from build123d import *

# Parameters (mm, degrees)
F1_DEPTH = 3


with BuildPart() as f1:
    # F0 (on Top) → F1 (new body)
    with BuildSketch(Plane.XY):
        Polygon((-34.93066, -38.541029), (-34.93066, 10.958971), (-52.43066, 10.958971), (-52.43066, 13.958971), (-67.43066, 13.958971), (-67.43066, 10.958971), (-84.93066, 10.958971), (-84.93066, -38.541029), (-87.93066, -38.541029), (-87.93066, -48.541029), (-84.93066, -48.541029), (-84.93066, -53.541029), (-82.93066, -53.541029), (-82.93066, -52.041029), (-80.43066, -52.041029), (-80.43066, -53.541029), (-77.43066, -53.541029), (-77.43066, -56.541029), (-80.43066, -56.541029), (-80.43066, -58.041029), (-82.93066, -58.041029), (-82.93066, -56.541029), (-84.93066, -56.541029), (-84.93066, -61.541029), (-87.93066, -61.541029), (-87.93066, -71.541029), (-84.93066, -71.541029), (-84.93066, -121.041029), (-67.43066, -121.041029), (-67.43066, -124.041029), (-52.43066, -124.041029), (-52.43066, -121.041029), (-34.93066, -121.041029), (-34.93066, -71.541029), (-31.93066, -71.541029), (-31.93066, -61.541029), (-34.93066, -61.541029), (-34.93066, -56.541029), (-36.93066, -56.541029), (-36.93066, -58.041029), (-39.43066, -58.041029), (-39.43066, -56.541029), (-42.43066, -56.541029), (-42.43066, -53.541029), (-39.43066, -53.541029), (-39.43066, -52.041029), (-36.93066, -52.041029), (-36.93066, -53.541029), (-34.93066, -53.541029), (-34.93066, -48.541029), (-31.93066, -48.541029), (-31.93066, -38.541029), align=None)
        with BuildLine():
            Line((-75.93066, -81.041029), (-43.93066, -81.041029))
            ThreePointArc((-43.93066, -81.041029), (-42.869999, -81.480369), (-42.43066, -82.541029))
            Line((-42.43066, -82.541029), (-42.43066, -109.541029))
            ThreePointArc((-42.43066, -109.541029), (-42.869999, -110.601689), (-43.93066, -111.041029))
            Line((-43.93066, -111.041029), (-75.93066, -111.041029))
            ThreePointArc((-75.93066, -111.041029), (-76.99132, -110.601689), (-77.43066, -109.541029))
            Line((-77.43066, -109.541029), (-77.43066, -82.541029))
            ThreePointArc((-77.43066, -82.541029), (-76.99132, -81.480369), (-75.93066, -81.041029))
        make_face(mode=Mode.SUBTRACT)
        with BuildLine():
            ThreePointArc((-77.43066, -0.541029), (-76.99132, 0.519631), (-75.93066, 0.958971))
            Line((-75.93066, 0.958971), (-43.93066, 0.958971))
            ThreePointArc((-43.93066, 0.958971), (-42.869999, 0.519631), (-42.43066, -0.541029))
            Line((-42.43066, -0.541029), (-42.43066, -27.541029))
            ThreePointArc((-42.43066, -27.541029), (-42.869999, -28.601689), (-43.93066, -29.041029))
            Line((-43.93066, -29.041029), (-75.93066, -29.041029))
            ThreePointArc((-75.93066, -29.041029), (-76.99132, -28.601689), (-77.43066, -27.541029))
            Line((-77.43066, -27.541029), (-77.43066, -0.541029))
        make_face(mode=Mode.SUBTRACT)
    extrude(amount=F1_DEPTH)


solid = f1.part
The model under review builds one solid part; all positions refer to its coordinate system, in mm. A direction names the side the tool comes from. Give positions to 0.01 mm unless a question says otherwise; leave off trailing zeros. Order: outer loops, then holes, each group sorted by start corner. A loop starts at its lowest first (then second) coordinate and runs counter-clockwise, first axis right, second up. Notation, with made-up numbers: M -29,18.5 L 1,18.5 A26 ccw 1,50.5 Z; hole C 34.25,45.25 d1. An arc over 180 degrees is marked long. Use one line per item in the form item = value. Start each with the question number.
Item 1: We need section D-D on z = 1.4. Give the number of separate pieces and of enclosed holes in the cut face, plus the area to 3 significant figures.
Item 2: To check wall thickness, follow line 1 along Y through (x, z) = (-51.5, 0.8); line 2 along Y through (x, z) = (-58.5, 1.8); line 3 along X through (y, z) = (-100.5, 2.4). State the ranges of each line that lie inside material, in increasing order. Write a range as from..to.
Item 3: We need section B-B on x = -74. Give the boundary of the cut face in (y, z), plus the area to 3 significant figures.
Item 4: The part is to be moulded in two halves that separate along Y. For faces 5 (the flat face through (-31.931, -67, 1)), 6 (the flat face through (-86, -61.541, 1)), 7 (the flat face through (-76, -121.041, 1)), say which applies: pulls with the +Y half, pulls with the -Y half, needs draft (parallel to the pull), parting line crosses it, or undercut.
Item 5: We need section A-A on y = -12.5. Give the boundary of the cut face in (x, z).
Item 6: Insertion check: pin 1 Ø1.5 at (x, z) = (-79, 1.5) entering from -Y; pin 2 Ø1.5 at (y, z) = (-60.5, 1) entering from -X; pin 3 Ø0.8 at (y, z) = (-53, 2) entering from +X. Each pin has a flat end and moves straight along its axis. Give the tip position at first contact, or say it passes through.
Item 7: For faces 1 (the flat face through (-76, 10.959, 1)), 2 (the flat face through (-79, -56.541, 1)), 3 (the flat face through (-38, -52.041, 1)), 4 (the flat face through (-33, -61.541, 1)), list the 3-axis set-ups (+Z, -Z, +X, -X, +Y, -Y) from which the entire face can be reached by the end or side of a thin tool; tool diameter is ignored.
Item 8: We need section C-C on x = -55.5. Give the boundary of the cut face in (y, z), plus the area to 3 significant figures.
Completed:
q1.separate_pieces = 1
q1.enclosed_holes = 2
q1.area = 4,650 mm²
q2.line_1 = -121.04..-111.04, -81.04..-29.04, 0.96..10.96
q2.line_2 = -124.04..-111.04, -81.04..-29.04, 0.96..13.96
q2.line_3 = -84.93..-77.43, -42.43..-34.93
q3.outline = M -121.04,0 L -111.04,0 L -111.04,3 L -121.04,3 Z; M -81.04,0 L -29.04,0 L -29.04,3 L -81.04,3 Z; M 0.96,0 L 10.96,0 L 10.96,3 L 0.96,3 Z
q3.area = 216 mm²
q4.face_5 = needs draft
q4.face_6 = undercut
q4.face_7 = pulls with the -Y half
q5.outline = M -84.93,0 L -77.43,0 L -77.43,3 L -84.93,3 Z; M -42.43,0 L -34.93,0 L -34.93,3 L -42.43,3 Z
q6.pin_1 = -121.04
q6.pin_2 = -84.93
q6.pin_3 = -34.93
q7.face_1 = +Z, -Z, -X, +Y
q7.face_2 = +Z, -Z, -X
q7.face_3 = +Z, -Z
q7.face_4 = +Z, -Z, +X
q8.outline = M -124.04,0 L -111.04,0 L -111.04,3 L -124.04,3 Z; M -81.04,0 L -29.04,0 L -29.04,3 L -81.04,3 Z; M 0.96,0 L 13.96,0 L 13.96,3 L 0.96,3 Z
q8.area = 234 mm²
